Geometry: see drawing. Coordinates: mm, zero at the bounding-box minimum. Coordinates: 2 decimals unless noted, no trailing zeros. Write each loop counter-clockwise with the first axis right and the second up, starting at its lowest first coordinate (ties: lowest second). Pieces come first, ordered by that corner, then holes. Notation, with made-up numbers: (41, 46.5) - (92, 46.5) arc R16 ccw to (92, 60.5) - close; hole circle Ø6 at (35.25, 43.5). An arc over 180 degrees is marked (long way). One line per question, with ' | ' between items. Start each with the question number.
Q1. Cut plane A-A, the plane z = 27.35. Return loops of the section in (x, y) (1 decimal), plus the area to 3 significant figures.
Q2. Cut plane D-D, the plane x = 18.5. Return loops of the section in (y, z) (1 decimal).
Q3. Cut plane B-B, the plane y = 22. Return loops of the section in (x, z) (1 decimal), plus the area to 3 significant figures.
Q4. Cut plane C-C, the plane z = 88. Return loops of the section in (x, y) (1 decimal), plus the area to 3 significant figures.
Q5. Draft query along X for the marked faces 1, 2, 3 and 4. Return one class per face: +X half, -X half, draft (parallel to the pull), parting line (faces both ways), or undercut.
Q6. Line query: line 1 (X direction, y = 24.25, z = 178) (1 decimal); line 2 (Y direction, x = 23.6, z = 10.35) (1 decimal); line 3 (Y direction, x = 23.35, z = 10.35) (1 decimal). Output: solid intervals per line, ascending.
Q7. Contact query for flat-ended pins moving along their axis: P1, Ø6, axis at x = 19, y = 16, coming from the +Z side; P2, Ø5, axis at x = 15, z = 109.5, coming from the +Y side (3 decimals). Output: stop coordinate, or through.
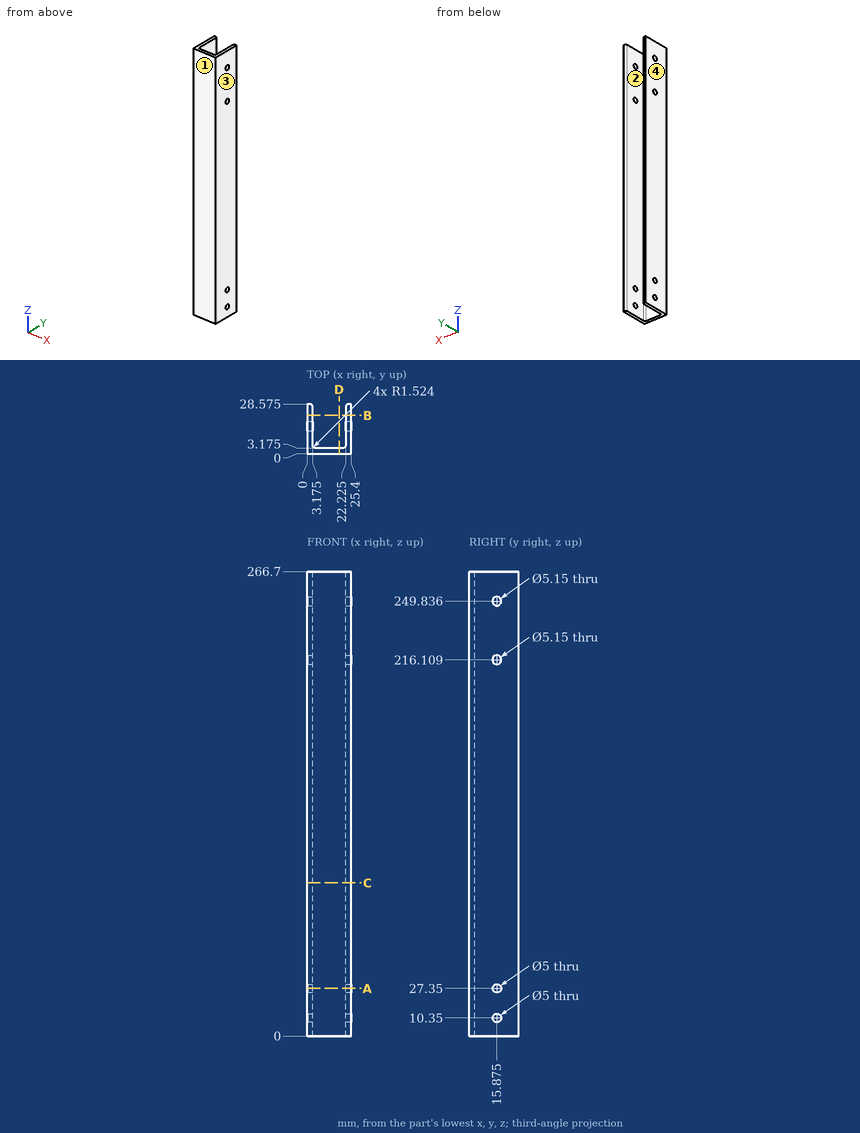
Reply:
1) outline: (0, 0) - (25.4, 0) - (25.4, 13.4) - (22.2, 13.4) - (22.2, 4.7) arc R1.5 cw to (20.7, 3.2) - (4.7, 3.2) arc R1.5 cw to (3.2, 4.7) - (3.2, 13.4) - (0, 13.4) - close; (0, 18.4) - (3.2, 18.4) - (3.2, 27.1) arc R1.5 ccw to (1.7, 28.6) - (0, 28.6) - close; (22.2, 18.4) - (25.4, 18.4) - (25.4, 28.6) - (23.7, 28.6) arc R1.5 ccw to (22.2, 27.1) - close | area: 210 mm^2
2) outline: (0, 0) - (3.2, 0) - (3.2, 266.7) - (0, 266.7) - close
3) outline: (0, 0) - (3.2, 0) - (3.2, 266.7) - (0, 266.7) - close; (22.2, 0) - (25.4, 0) - (25.4, 266.7) - (22.2, 266.7) - close | area: 1,690 mm^2
4) outline: (0, 0) - (25.4, 0) - (25.4, 28.6) - (23.7, 28.6) arc R1.5 ccw to (22.2, 27.1) - (22.2, 4.7) arc R1.5 cw to (20.7, 3.2) - (4.7, 3.2) arc R1.5 cw to (3.2, 4.7) - (3.2, 27.1) arc R1.5 ccw to (1.7, 28.6) - (0, 28.6) - close | area: 242 mm^2
5) face 1: draft | face 2: undercut | face 3: +X half | face 4: -X half
6) line 1: x = 0 to 3.2, 22.2 to 25.4 | line 2: y = 0 to 13.4, 18.4 to 28.6 | line 3: y = 0 to 13.4, 18.4 to 28.5
7) P1: passes through | P2: stops at y = 3.175
